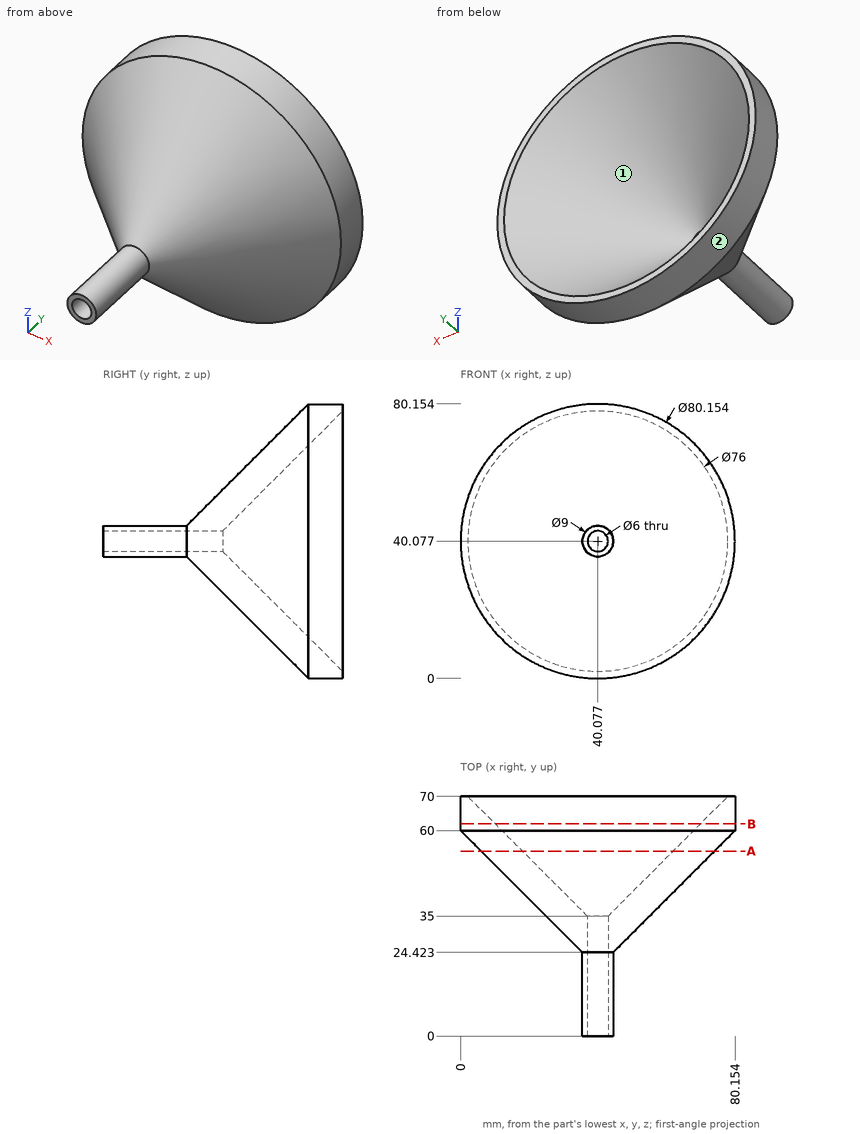
Can you work these out from the drawing? Everything is in mm from the part's minimum corner. Round coordinates to 2 decimals unless told otherwise and drop trailing zeros. Order: outer loops, then holes, each group sorted by start corner. A loop starts at its lowest first (then second) coordinate and runs counter-clockwise, first axis right, second up. Notation, with made-up numbers: (45.5, -20) -> (88.5, -20) arc R18 ccw to (88.5, -8) -> close; hole circle Ø11 at (14.5, 76). An arc over 180 degrees is marked (long way). Return JSON: item names as keys, results as strings. Group by question number.
1. I need wall thicknesses on line 1 (X direction, y = 64, z = 38.5); line 2 (X direction, y = 60, z = 21.5); line 3 (Y direction, x = 11.5, z = 30). Which ranges of each line are inside material? Lowest first, please. Write a range as [from, to].
2. If we section it at A-A, the plane y = 54: Write out the boundary of the cut face in (x, z), then the cut area to 3 significant figures.
3. Will these pins go through, and if not, where does the flat tip stop? pin 1 (9.5 mm diameter, centred on x = 40.08, z = 40.08, fed in from -Y); pin 2 (12 mm diameter, centred on y = 20, z = 43.5, fed in from -X); pin 3 (10 mm diameter, centred on y = 37.5, z = 57.5, fed in from +X); pin 4 (10 mm diameter, centred on x = 36.5, z = 39, fed in from +Y).
4. We'd pull the mould along Z, two halves only. Please class the marked faces 1 and 2: released by +Z, released by -Z, zero draft, split by the parting line, or undercut.
5. If we section it at B-B, the plane y = 62: Write out the boundary of the cut face in (x, z).
Output values:
{
 "1": {"line 1": "[0.03, 8.12], [72.04, 80.12]", "line 2": "[4.57, 19.13], [61.03, 75.59]", "line 3": "[50.22, 62.3]"},
 "2": {"outline": "circle Ø68.15 at (40.08, 40.08); hole circle Ø44 at (40.08, 40.08)", "area": "2,130 mm²"},
 "3": {"pin 1": "y = 0", "pin 2": "x = 34.51", "pin 3": "x = 56.14", "pin 4": "y = 40.74"},
 "4": {"face 1": "undercut", "face 2": "split by the parting line"},
 "5": {"outline": "circle Ø80.15 at (40.08, 40.08); hole circle Ø60 at (40.08, 40.08)"}
}
